```python
from build123d import *

# Parameters (mm, degrees)
SKETCH_1_W          = 150
SKETCH_1_H          = 110
EXTRUDE_1_DEPTH     = 35
FILLET_1_R          = 10
SKETCH_4_R          = 2
CUT_EXTRUDE_1_DEPTH = 2
CUT_EXTRUDE_2_DEPTH = 2


with BuildPart() as part:
    # Sketch 1 → Extrude 1 (new body)
    with BuildSketch(Plane.XY):
        Rectangle(SKETCH_1_W, SKETCH_1_H)
    extrude(amount=EXTRUDE_1_DEPTH)

    # Fillet 1
    fillet_1_edges = [part.edges().sort_by_distance(p)[0] for p in [
        (0, 55, 0),
        (75, 0, 0),
        (0, -55, 0),
        (-75, 0, 0),
    ]]
    fillet(fillet_1_edges, radius=FILLET_1_R)

    # Sketch 4 → Cut-Extrude 1 (cut)
    with BuildSketch(Plane.XY.offset(35)):
        with Locations((-66, 32)):
            Circle(SKETCH_4_R)
        with Locations(Location((-66, -19, 0), (0, 0, 180))):
            Circle(SKETCH_4_R)
        with Locations((66, -19)):
            Circle(SKETCH_4_R)
        with Locations(Location((66, 32, 0), (0, 0, 180))):
            Circle(SKETCH_4_R)
    extrude(amount=-CUT_EXTRUDE_1_DEPTH, mode=Mode.SUBTRACT)

    # Sketch 5 → Cut-Extrude 2 (cut)
    with BuildSketch(Plane(origin=(0, 55, 0), x_dir=(1, 0, 0), z_dir=(0, 1, 0))):
        with BuildLine():
            Line((-6.5, -22.7), (6.5, -22.7))
            Line((6.5, -22.7), (6.5, -29.2))
            ThreePointArc((6.5, -29.2), (5.914213562, -30.614213562), (4.5, -31.2))
            Line((4.5, -31.2), (-4.5, -31.2))
            ThreePointArc((-4.5, -31.2), (-5.914213562, -30.614213562), (-6.5, -29.2))
            Line((-6.5, -29.2), (-6.5, -22.7))
        make_face()
        with BuildLine():
            Line((16.5, -22.7), (29.5, -22.7))
            Line((29.5, -22.7), (29.5, -29.2))
            ThreePointArc((29.5, -29.2), (28.914213562, -30.614213562), (27.5, -31.2))
            Line((27.5, -31.2), (18.5, -31.2))
            ThreePointArc((18.5, -31.2), (17.085786438, -30.614213562), (16.5, -29.2))
            Line((16.5, -29.2), (16.5, -22.7))
        make_face()
        with BuildLine():
            Line((39.5, -22.7), (52.5, -22.7))
            Line((52.5, -22.7), (52.5, -29.2))
            ThreePointArc((52.5, -29.2), (51.914213562, -30.614213562), (50.5, -31.2))
            Line((50.5, -31.2), (41.5, -31.2))
            ThreePointArc((41.5, -31.2), (40.085786438, -30.614213562), (39.5, -29.2))
            Line((39.5, -29.2), (39.5, -22.7))
        make_face()
        with BuildLine():
            Line((-29.5, -22.7), (-16.5, -22.7))
            Line((-16.5, -22.7), (-16.5, -29.2))
            ThreePointArc((-16.5, -29.2), (-17.085786438, -30.614213562), (-18.5, -31.2))
            Line((-18.5, -31.2), (-27.5, -31.2))
            ThreePointArc((-27.5, -31.2), (-28.914213562, -30.614213562), (-29.5, -29.2))
            Line((-29.5, -29.2), (-29.5, -22.7))
        make_face()
    extrude(amount=-CUT_EXTRUDE_2_DEPTH, mode=Mode.SUBTRACT)


solid = part.part
```
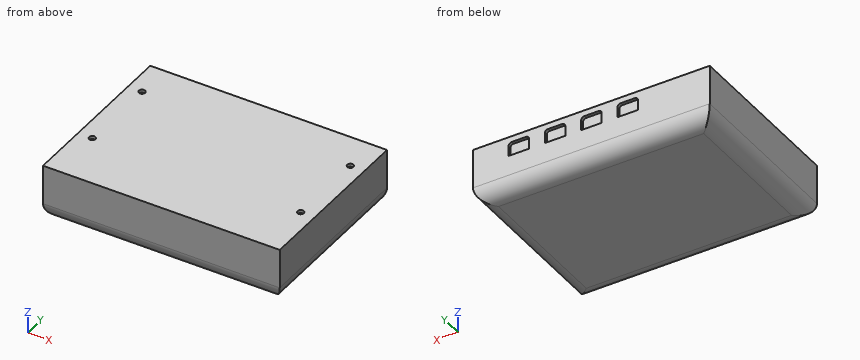
Can you work these out from the model? Positions are in its coordinate system, mm. Give positions to 0.01 mm unless a question says otherwise; leave off trailing zeros. Order: outer loops, then holes, each group sorted by start corner. A loop starts at its lowest first (then second) coordinate and runs counter-clockwise, first axis right, second up. Notation, with made-up numbers: M 32.25,13 L 87.25,13 A29 cw 87.25,33 Z; hole C -14.5,-31 d6. An arc over 180 degrees is marked long. Write item = value, one per line. Start each with the question number.
Q1. I need wall thicknesses on probe 1 along Y at (x, z) = (-66, 34.55); probe 2 along Z at (x, y) = (69.5, 17); probe 3 along Y at (x, z) = (10, 8). Which ranges of each line are inside material? Lowest first, please. Write a range as [from, to].
Q2. Suppose I cut it at A-A (x = 46). Write out the boundary of the cut face in (y, z), plus the area to 3 significant figures.
Q3. Will this pin go through, and if not, where does the flat tip stop? pin 1 Ø1.2 at (x, y) = (-66, -20) entering from +Z.
Check result:
q1.probe_1 = [-55, -21], [-17, 30], [34, 55]
q1.probe_2 = [1.07, 35]
q1.probe_3 = [-54.8, 54.8]
q2.outline = M -55,10 A10 ccw -45,0 L 45,0 A10 ccw 55,10 L 55,22.7 L 53,22.7 L 53,31.2 L 55,31.2 L 55,35 L -55,35 Z
q2.area = 3,790 mm2
q3.pin_1 = 33
